The listing builds one solid part. Answer for the finished solid, in the listing's coordinates (mm). A direction names the side the tool comes from. Round coordinates to 2 decimals unless told otherwise and drop trailing zeros. Write each loop counter-clockwise with the first axis right and the second up, starting at its lowest first coordinate (ties: lowest second). Pieces come first, ordered by that corner, then holes.
from build123d import *

# Parameters (mm, degrees)
F0_W     = 60.2390449494
F0_H     = 45.3361533582
F1_DEPTH = 72.3
F2_T     = -2.5


with BuildPart() as f1:
    # F0 (on Front) → F1 (new body)
    with BuildSketch(Plane.XZ):
        with BuildLine():
            add(Edge.make_bspline(
                [(-29.0998518467, 45.3361533582), (-30.3761818728, 33.0718928085), (-29.7380168597, 16.5359464043), (-29.0998518467, 0)],
                knots=[0.4101722166, 0.4101722166, 0.4101722166, 0.4101722166, 1, 1, 1, 1], degree=3))
            Line((-29.0998518467, 0), (-29.0998518467, 45.3361533582))
        make_face()
        with BuildLine():
            Line((31.1391931027, 45.3361533582), (31.1391931027, 0))
            add(Edge.make_bspline(
                [(31.1391931027, 45.3361533582), (32.2873652792, 33.0616785906), (31.713279191, 16.5308392953), (31.1391931027, 0)],
                knots=[0.4096689576, 0.4096689576, 0.4096689576, 0.4096689576, 1, 1, 1, 1], degree=3))
        make_face()
        with Locations((1.019670628, 22.6680766791)):
            Rectangle(F0_W, F0_H)
        with BuildLine():
            add(Edge.make_bspline(
                [(-24.5854519308, 66.7906925082), (-26.3988654728, 60.3277684568), (-28.2122790148, 53.8648444053), (-29.0998518467, 45.3361533582)],
                knots=[0, 0, 0, 0, 0.4101722166, 0.4101722166, 0.4101722166, 0.4101722166], degree=3))
            Line((-29.0998518467, 45.3361533582), (31.1391931027, 45.3361533582))
            add(Edge.make_bspline(
                [(27.0899850875, 66.7906925082), (28.7161935637, 60.3224495827), (30.3424020399, 53.8542066572), (31.1391931027, 45.3361533582)],
                knots=[0, 0, 0, 0, 0.4096689576, 0.4096689576, 0.4096689576, 0.4096689576], degree=3))
            Line((27.0899850875, 66.7906925082), (0, 66.7906925082))
            Line((0, 66.7906925082), (-21.6005891562, 66.7906925082))
            Line((-21.6005891562, 66.7906925082), (-24.5854519308, 66.7906925082))
        make_face()
    extrude(amount=F1_DEPTH)

    # F2
    f2_openings = [f1.faces().sort_by_distance(p)[0] for p in [
        (1.031904, -72.3, 32.779225),
    ]]
    offset(amount=F2_T, openings=f2_openings, kind=Kind.INTERSECTION)


solid = f1.part
1. Given pin 1 (8 mm diameter, centred on y = -11.5, z = 47.5, fed in from -X); pin 2 (12 mm diameter, centred on y = -43, z = 19, fed in from -X); pin 3 (8 mm diameter, centred on y = -34.5, z = 51.5, fed in from -X), each flat-ended and moving along its own axis, determine where each tip first touches the part or whether it passes through.
Geometry says:
pin 1: stops at x = -29.27
pin 2: stops at x = -29.82
pin 3: stops at x = -28.85
2. Section A-A on x = 16 is taken. Determine the outline of the cut face in (y, z), plus the area to 3 significant figures.
Geometry says:
outline: (-72.3, 0) - (0, 0) - (0, 66.79) - (-72.3, 66.79) - (-72.3, 64.29) - (-2.5, 64.29) - (-2.5, 2.5) - (-72.3, 2.5) - close
area: 516 mm2
3. A tool of negligible diameter and unlimited length cuts with its end or side. For faces 1 (the face through (1, -37, 2.5)), 2 (the face through (1, -36, 0)), from which of +Z, -Z, +X, -X, +Y, -Y can it reach the whole face along a straight path? Write none if from no direction.
Geometry says:
face 1: -Y
face 2: -Z, +X, -X, +Y, -Y
4. Straight lines are drawn through the part: line 1 along Z through (x, y) = (8, -12.5); line 2 along X through (y, z) = (-67.5, 31); line 3 along Y through (x, z) = (0, 48.5). For each, find the intervals that lie inside material, in ascending order.
Geometry says:
line 1: z = 0 to 2.5, 64.29 to 66.79
line 2: x = -29.82 to -27.32, 29.29 to 31.79
line 3: y = -2.5 to 0
5. For a pull along X with two mould halves and no side action, classify faces 3 (the face through (2, -36, 66.791)), 4 (the face through (2, -37, 64.291)) as released by +X, released by -X, zero draft, split by the parting line, or undercut.
Geometry says:
face 3: zero draft
face 4: undercut
